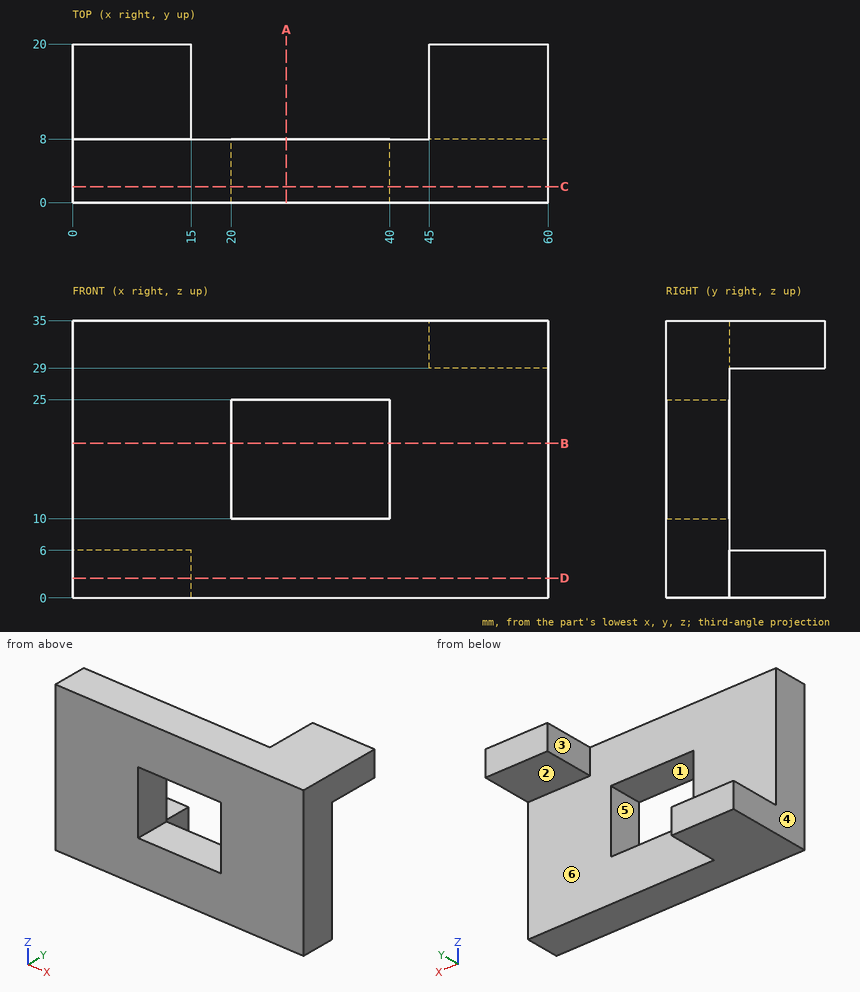
Study the drawing (mm; zero at the part's minimum x, y, z) and answer. A direction names the side the tool comes from. Coordinates: 2 decimals unless noted, no trailing zeros. Write each loop counter-clockwise with the first axis right and the second up, starting at its lowest first coordinate (ties: lowest second). Pieces come first, ordered by that corner, then holes. Notation, with made-up numbers: (81.5, 48.5) - (93.5, 48.5) arc R33 ccw to (93.5, 87.5) - close; hole circle Ø2 at (20, 39). An arc over 180 degrees is marked (long way). One line per question, with ' | ' between items.
1) Flat-ended cylindrical pins translate along their axes: P1, Ø9.5, axis at x = 51.5, y = 15.5, coming from the -Z side; P2, Ø9.5, axis at x = 10, y = 16, coming from the +Z side; P3, Ø5, axis at x = 41, z = 8.5, coming from the +Y side. Find the tip coordinate at first contact, or state that the pin passes through.
Checks:
P1: z = 29 | P2: z = 6 | P3: y = 8
2) Consider probe 1 along X at (y, z) = (3.5, 23); probe 2 along Z at (x, y) = (23.5, 4.25); probe 3 along Y at (x, z) = (12.5, 7.5). Determine where each line is inside the solid, lowest interval first. Write a range as [from, to].
Checks:
probe 1: [0, 20], [40, 60] | probe 2: [0, 10], [25, 35] | probe 3: [0, 8]
3) Find section C-C, the plane y = 2. Determine the outline of the cut face in (x, z), and give its area (3 significant figures).
Checks:
outline: (0, 0) - (60, 0) - (60, 35) - (0, 35) - close; hole (20, 10) - (40, 10) - (40, 25) - (20, 25) - close | area: 1,800 mm2
4) For the marked faces 1, 2 and 3, determine the directions among +Z, -Z, +X, -X, +Y, -Y from which every point of the face is accessible in a straight line to the end or side of a thin tool.
Checks:
face 1: +Y, -Y | face 2: -Z, +X, -X, +Y | face 3: +Z, -Z, -X, +Y
5) Find section A-A, the plane x = 27. Determine the outline of the cut face in (y, z), and give its area (3 significant figures).
Checks:
outline: (0, 0) - (8, 0) - (8, 10) - (0, 10) - close; (0, 25) - (8, 25) - (8, 35) - (0, 35) - close | area: 160 mm2
6) The mould has two halves that part along X. Classify the marked faces 4, 5 and 6: +X half, -X half, draft (parallel to the pull), parting line (faces both ways), or undercut.
Checks:
face 4: -X half | face 5: undercut | face 6: draft
7) Find section D-D, the plane z = 2.5. Determine the outline of the cut face in (x, y), and give its area (3 significant figures).
Checks:
outline: (0, 0) - (60, 0) - (60, 8) - (15, 8) - (15, 20) - (0, 20) - close | area: 660 mm2
8) Find section B-B, the plane z = 19.5. Determine the outline of the cut face in (x, y), and give its area (3 significant figures).
Checks:
outline: (0, 0) - (20, 0) - (20, 8) - (0, 8) - close; (40, 0) - (60, 0) - (60, 8) - (40, 8) - close | area: 320 mm2
